For this review, take the finished solid that the model builds, in its own axes (mm). A direction names the side the tool comes from. Coordinates: 2 decimals unless noted, no trailing zeros. Write each loop counter-clockwise with the first axis right and the second up, starting at its lowest first coordinate (ties: lowest second). Pieces come first, ordered by that corner, then holes.
```python
from build123d import *


with BuildPart() as f1:
    # F0 (on Front) → F1 (revolve)
    with BuildSketch(Plane.XZ):
        with BuildLine():
            Line((-2.25, 49.230757), (-13, 49.230757))
            Line((-13, 49.230757), (-13, 47.630757))
            Line((-13, 47.630757), (-11.4, 47.630757))
            Line((-11.4, 47.630757), (-11.4, 46.030757))
            Line((-11.4, 46.030757), (-13, 46.030757))
            Line((-13, 46.030757), (-13, 43.030757))
            ThreePointArc((-13, 43.030757), (-6.166339, 8.630757), (-13, -25.769243))
            Line((-13, -25.769243), (-13, -30.769243))
            Line((-13, -30.769243), (0, -30.769243))
            Line((0, -30.769243), (0, 50.830757))
            Line((0, 50.830757), (-2.25, 50.830757))
            Line((-2.25, 50.830757), (-2.25, 49.230757))
        make_face()
    revolve(axis=Axis((0, 0, 10.030757), (0, 0, -1)))


solid = f1.part
```
1) For L1, parallel to Z at x = -10.25, y = -6.5; L2, parallel to Z at x = 4.75, y = 3; L3, parallel to X at y = -2.75, z = 46.5, list the stretches that pass through material, from the lowest coordinate up.
2) Consider section D-D (z = 10). Give the boundary of the cut face in (x, y), then the cut area to 3 significant figures.
3) The part is to be moulded in two halves that separate along Z. For faces 1 (the face through (0, 0, 50.831)), 2 (the face through (-8, -9, 47.631)), 3 (the face through (0.29, 2.23, 50.02)), say which applies: pulls with the +Z half, pulls with the -Z half, needs draft (parallel to the pull), parting line crosses it, or undercut.
4) Tool access review of faces 4 (the face through (9, -7, 47)), 5 (the face through (10.316, -7.91, 48.42)): name each direction out of +Z, -Z, +X, -X, +Y, -Y from which nothing blocks a thin tool from reaching the whole face with its end or side.
5) Consider section A-A (y = 0). Give the boundary of the cut face in (x, z), then the cut area to 3 significant figures.
6) Consider section C-C (z = -3). Give the boundary of the cut face in (x, y), then the cut area to 3 significant figures.
7) Clearance check with flat-ended pins moving along their axes: P1, Ø6, axis at y = -5.5, z = 40.5, coming from the -X side; P2, Ø2, axis at y = 9, z = 24.5, coming from the +X side; P3, Ø6, axis at x = -5, z = -18.5, coming from the -Y side; P4, Ø1.5, axis at x = 6.5, z = 23.5, coming from the -Y side. State where each tip first meets the part, or that it passes through.
Results:
1. L1: z = -30.77 to -23.6, 40.87 to 46.03, 47.63 to 49.23
1. L2: z = -30.77 to 49.23
1. L3: x = -11.06 to 11.06
2. outline: circle Ø12.35 at (0, 0)
2. area: 120 mm2
3. face 1: pulls with the +Z half
3. face 2: undercut
3. face 3: needs draft
4. face 4: none
4. face 5: +Z, -Z
5. outline: (-13, -30.77) - (13, -30.77) - (13, -25.77) arc R90 cw to (13, 43.03) - (13, 46.03) - (11.4, 46.03) - (11.4, 47.63) - (13, 47.63) - (13, 49.23) - (2.25, 49.23) - (2.25, 50.83) - (-2.25, 50.83) - (-2.25, 49.23) - (-13, 49.23) - (-13, 47.63) - (-11.4, 47.63) - (-11.4, 46.03) - (-13, 46.03) - (-13, 43.03) arc R90 cw to (-13, -25.77) - close
5. area: 1,450 mm2
6. outline: circle Ø13.84 at (0, 0)
6. area: 150 mm2
7. P1: stops at x = -12.41
7. P2: passes through
7. P3: stops at y = -10.68
7. P4: stops at y = -4.68
